Geometry check sheet. Reference: the model listing, model coordinates, mm. A direction names the side the tool comes from. Coordinates: 2 decimals unless noted, no trailing zeros. Write each loop counter-clockwise with the first axis right and the second up, starting at its lowest first coordinate (ties: lowest second). Pieces come first, ordered by that corner, then holes. Notation, with made-up numbers: (56.25, -0.75) -> (100.25, -0.75) arc R14 ccw to (100.25, 10.25) -> close; hole circle Ø11 at (-37, 42.5). An arc over 180 degrees is marked (long way). Put each result on its own line as item: value. Start each with the question number.
from build123d import *

# Parameters (mm, degrees)
F0_W      = 47.5
F0_H      = 35
F1_DEPTH  = 7.5
F2_W      = 10
F2_H      = 35
F3_DEPTH  = 10
F5_DEPTH  = 10.001
F7_DEPTH  = 7.501
F9_DEPTH  = 7.501
F10_W     = 22.5
F10_H     = 4
F11_DEPTH = 7.501


with BuildPart() as f1:
    # F0 (on Top) → F1 (new body)
    with BuildSketch(Plane.XY):
        with Locations((8.500643, -14.324561)):
            Rectangle(F0_W, F0_H)
    extrude(amount=F1_DEPTH)

    # F2 (on face) → F3 (join)
    with BuildSketch(Plane.XY.offset(7.5)):
        with Locations((-10.249357, -14.324561)):
            Rectangle(F2_W, F2_H)
    extrude(amount=F3_DEPTH)

    # F4 (on face) → F5 (cut, through all)
    with BuildSketch(Plane.YZ.offset(-5.249357)):
        Polygon((-1.824561, 12.5), (-4.324561, 17.5), (-24.324561, 17.5), (-26.824561, 12.5), align=None)
    extrude(amount=-F5_DEPTH, mode=Mode.SUBTRACT)

    # F6 (on face) → F7 (cut, through all)
    with BuildSketch(Plane.XY.offset(7.5)):
        Polygon((19.750643, -31.824561), (32.250643, -31.824561), (32.250643, -18.824561), align=None)
    extrude(amount=-F7_DEPTH, mode=Mode.SUBTRACT)

    # F8 (on face) → F9 (cut, through all)
    with BuildSketch(Plane.XY.offset(7.5)):
        Polygon((19.750643, 3.175439), (32.250643, -7.824561), (32.250643, 3.175439), align=None)
    extrude(amount=-F9_DEPTH, mode=Mode.SUBTRACT)

    # F10 (on face) → F11 (cut, through all)
    with BuildSketch(Plane.XY.offset(7.5)):
        with Locations((21.000643, -14.324561)):
            Rectangle(F10_W, F10_H)
    extrude(amount=-F11_DEPTH, mode=Mode.SUBTRACT)


solid = f1.part
Item 1: Section check A-A, the plane x = 18. Enter the section's corners in (y, z).
Item 2: Go/stop test with flat-tipped pins: P1, Ø6, axis at x = 25.5, z = 7.5, coming from the -Y side; P2, Ø3, axis at y = -14.5, z = 4, coming from the +X side; P3, Ø4, axis at x = 22, z = 2.5, coming from the +Y side; P4, Ø1.5, axis at x = 26.5, y = -22, coming from the -Z side. Record where each tip stops, or that it passes through.
Item 3: Section check B-B, the plane z = 13.75. Enter the section's corners in (x, y).
Item 4: Section check C-C, the plane y = -9. Enter the section's corners in (x, z), and give its area (3 significant figures).
Item 5: Scan lines: line 1 along X through (y, z) = (-10, 11.25); line 2 along Z through (x, y) = (3.5, -3.5); line 3 along Z through (x, y) = (-6, -26). Record each from-to range of solid material in increasing order. Write a range as [from, to].
Item 6: Section check D-D, the plane z = 5.75. Enter the section's corners in (x, y).
Item 7: Access from +Z, -Z, +X, -X, +Y, -Y to the whole of each face (thin tool, end or side, straight path). Record for faces 1 (the flat face through (-10.179, -25.557, 15.035)), 2 (the flat face through (9, -14, 7.5)), 3 (the flat face through (9.751, -14, 4)).
Item 8: Mould release check, pull along Y, two halves, no side actions. Record for faces 4 (the flat face through (21, -12.325, 4)), 5 (the flat face through (-15.249, -15, 7)), 6 (the flat face through (25.913, -2.248, 3.802)): released by +Y, released by -Y, zero draft, split by the parting line, or undercut.
From the geometry:
1. outline: (-31.82, 0) -> (-16.32, 0) -> (-16.32, 7.5) -> (-31.82, 7.5) -> close; (-12.32, 0) -> (3.18, 0) -> (3.18, 7.5) -> (-12.32, 7.5) -> close
2. P1: y = -28.97
2. P2: x = 9.75
2. P3: y = 2.96
2. P4: z = 0
3. outline: (-15.25, -31.82) -> (-5.25, -31.82) -> (-5.25, -26.2) -> (-15.25, -26.2) -> close; (-15.25, -2.45) -> (-5.25, -2.45) -> (-5.25, 3.18) -> (-15.25, 3.18) -> close
4. outline: (-15.25, 0) -> (32.25, 0) -> (32.25, 7.5) -> (-5.25, 7.5) -> (-5.25, 12.5) -> (-15.25, 12.5) -> close
4. area: 406 mm²
5. line 1: [-15.25, -5.25]
5. line 2: [0, 7.5]
5. line 3: [0, 12.5], [14.15, 17.5]
6. outline: (-15.25, -31.82) -> (19.75, -31.82) -> (32.25, -18.82) -> (32.25, -16.32) -> (9.75, -16.32) -> (9.75, -12.32) -> (32.25, -12.32) -> (32.25, -7.82) -> (19.75, 3.18) -> (-15.25, 3.18) -> close
7. face 1: +X, -X
7. face 2: +Z, +X, +Y, -Y
7. face 3: +Z, -Z, +X
8. face 4: undercut
8. face 5: zero draft
8. face 6: released by +Y
